Verification items for the finished model (mm, model axes). A direction names the side the tool comes from. Coordinates: 2 decimals unless noted, no trailing zeros. Write each loop counter-clockwise with the first axis right and the second up, starting at its lowest first coordinate (ties: lowest second). Pieces come first, ordered by that corner, then holes. Notation, with made-up numbers: M 74.25,40.25 L 95.25,40.25 A38 cw 95.25,78.25 Z; hole C -5,26 d1. An arc over 180 degrees is marked long. One line per item, written item: value.
```python
from build123d import *

# Parameters (mm, degrees)
SKETCH1_W           = 60
SKETCH1_H           = 20
BOSS_EXTRUDE1_DEPTH = 10
SKETCH2_R           = 1
CUT_EXTRUDE1_DEPTH  = 10
CUT_EXTRUDE4_DEPTH  = 34.166247904
SKETCH6_R           = 1.5
CUT_EXTRUDE5_DEPTH  = 46.82575695
CUT_EXTRUDE6_START  = -5
SKETCH7_R           = 3.5
CUT_EXTRUDE6_DEPTH  = 41.82575695
FILLET2_R           = 2


with BuildPart() as part:
    # Sketch1 → Boss-Extrude1 (new body)
    with BuildSketch(Plane(origin=(0, 0, 0), x_dir=(1, 0, 0), z_dir=(0, 1, 0))):
        Rectangle(SKETCH1_W, SKETCH1_H)
    extrude(amount=BOSS_EXTRUDE1_DEPTH)

    # Sketch2 → Cut-Extrude1 (cut)
    with BuildSketch(Plane(origin=(0, 10, 0), x_dir=(1, 0, 0), z_dir=(0, 1, 0))):
        with Locations(Location((-25, 4.25, 0), (0, 0, 270))):
            Circle(SKETCH2_R)
        with Locations(Location((-16.5, 4.25, 0), (0, 0, 270))):
            Circle(SKETCH2_R)
        with Locations(Location((-16.5, -4.25, 0), (0, 0, 270))):
            Circle(SKETCH2_R)
        with Locations(Location((-25, -4.25, 0), (0, 0, 270))):
            Circle(SKETCH2_R)
    extrude(amount=-CUT_EXTRUDE1_DEPTH, mode=Mode.SUBTRACT)

    # Sketch5 → Cut-Extrude4 (cut, through all)
    with BuildSketch(Plane(origin=(0, 10, 0), x_dir=(1, 0, 0), z_dir=(0, 1, 0))):
        Polygon((10, -10), (30, 10), (30, -10), align=None)
    extrude(amount=-CUT_EXTRUDE4_DEPTH, mode=Mode.SUBTRACT)

    # Sketch6 → Cut-Extrude5 (cut, through all)
    with BuildSketch(Plane(origin=(10, 0, 10), x_dir=(0.7071067811865487, 0, -0.7071067811865464), z_dir=(0.7071067811865464, 0, 0.7071067811865487))):
        with Locations((19, 5)):
            Circle(SKETCH6_R)
        with Locations((9, 5)):
            Circle(SKETCH6_R)
    extrude(amount=-CUT_EXTRUDE5_DEPTH, mode=Mode.SUBTRACT)

    # Sketch7 → Cut-Extrude6 (cut, through all)
    with BuildSketch(Plane(origin=(10, 0, 10), x_dir=(0.7071067811865487, 0, -0.7071067811865464), z_dir=(0.7071067811865464, 0, 0.7071067811865487)).offset(CUT_EXTRUDE6_START)):
        with Locations((19, 5)):
            Circle(SKETCH7_R)
        with Locations((9, 5)):
            Circle(SKETCH7_R)
    extrude(amount=-CUT_EXTRUDE6_DEPTH, mode=Mode.SUBTRACT)

    # Fillet2
    # the kernel refuses this fillet: 2 mm, written as the material it takes off along each edge
    with BuildSketch(Plane(origin=(15, 10, 10), x_dir=(0, -1, 0), z_dir=(-1, 0, 0))) as fillet2_piece_1:
        with BuildLine():
            CenterArc((FILLET2_R, -FILLET2_R), FILLET2_R, 90, 90)
            Line((0, -FILLET2_R), (0, 0))
            Line((0, 0), (FILLET2_R, 0))
        make_face()
    extrude(amount=50, mode=Mode.SUBTRACT)
    with BuildSketch(Plane(origin=(15, 0, 10), x_dir=(0, 1, 0), z_dir=(-1, 0, 0))) as fillet2_piece_2:
        with BuildLine():
            CenterArc((FILLET2_R, FILLET2_R), FILLET2_R, 180, 90)
            Line((0, FILLET2_R), (0, 0))
            Line((0, 0), (FILLET2_R, 0))
        make_face()
    extrude(amount=50, mode=Mode.SUBTRACT)
    with BuildSketch(Plane(origin=(-35, 0, -10), x_dir=(0, 0, 1), z_dir=(1, 0, 0))) as fillet2_piece_3:
        with BuildLine():
            CenterArc((FILLET2_R, -FILLET2_R), FILLET2_R, 90, 90)
            Line((0, -FILLET2_R), (0, 0))
            Line((0, 0), (FILLET2_R, 0))
        make_face()
    extrude(amount=70, mode=Mode.SUBTRACT)
    with BuildSketch(Plane(origin=(-35, 10, -10), x_dir=(0, 0, 1), z_dir=(1, 0, 0))) as fillet2_piece_4:
        with BuildLine():
            CenterArc((FILLET2_R, FILLET2_R), FILLET2_R, 180, 90)
            Line((0, FILLET2_R), (0, 0))
            Line((0, 0), (FILLET2_R, 0))
        make_face()
    extrude(amount=70, mode=Mode.SUBTRACT)


solid = part.part
```
Item 1: Access from +Z, -Z, +X, -X, +Y, -Y to the whole of each face (thin tool, end or side, straight path). Record for faces 4 (the face through (20.965, 4.271, -8.036)), 5 (the face through (-25.976, 5.07, -4.467)).
The answers:
face 4: none
face 5: +Y, -Y
Item 2: Scan lines: line 1 (X direction, y = 3, z = -7.75); line 2 (X direction, y = 4, z = 3.75); line 3 (X direction, y = 5.5, z = -5). Record each from-to range of solid material in increasing order.
The answers:
line 1: x = -30 to 0.92, 9.04 to 15.06, 20.68 to 27.75
line 2: x = -30 to -25.87, -24.13 to -17.37, -15.63 to 14.9
line 3: x = -30 to -25.66, -24.34 to -17.16, -15.84 to 2.83, 12.63 to 16.97, 17.93 to 19.87, 23.87 to 25
Item 3: Draft check along Y on faces 1 (the face through (15.63, 5.45, 0.88)), 2 (the face through (-8, 10, 0)), 3 (the face through (-25.976, 5.07, 4.033)). Enter one of: released by +Y, released by -Y, zero draft, split by the parting line, or undercut.
The answers:
face 1: undercut
face 2: released by +Y
face 3: zero draft
Item 4: Cross-section at A-A, the plane x = -16.5. Enter the section's corners in (y, z).
The answers:
outline: M 0,-8 A2 ccw 2,-10 L 8,-10 A2 ccw 10,-8 L 10,-5.25 L 0,-5.25 Z; M 0,-3.25 L 10,-3.25 L 10,3.25 L 0,3.25 Z; M 0,5.25 L 10,5.25 L 10,8 A2 ccw 8,10 L 2,10 A2 ccw 0,8 Z
Item 5: Go/stop test with flat-tipped pins: P1, Ø1.5, axis at x = -6, y = 1, coming from the +Z side; P2, Ø2, axis at x = 6, y = 6, coming from the -Z side; P3, Ø1, axis at x = 13.5, y = 2.5, coming from the +Z side; P4, Ø1.2, axis at x = -25, z = -4.25, coming from the +Y side. Record where each tip stops, or that it passes through.
The answers:
P1: stops at z = 9.98
P2: stops at z = -3.13
P3: stops at z = 7
P4: passes through
Item 6: Cross-section at B-B, the plane y = 4.25. Enter the section's corners in (x, z), and give its area (3 significant figures).
The answers:
outline: M -30,-10 L -2.11,-10 L 10.41,2.52 L 11.91,1.02 L 15.45,4.55 L 10,10 L -30,10 Z; M 7.56,-10 L 12.04,-10 L 17.48,-4.55 L 18.98,-6.05 L 22.52,-2.52 L 17.28,2.72 L 13.75,-0.82 L 15.25,-2.32 Z; M 20.82,-7.89 L 22.32,-9.39 L 21.7,-10 L 30,-10 L 24.35,-4.35 Z; hole C -25,-4.25 d2; hole C -25,4.25 d2; hole C -16.5,-4.25 d2; hole C -16.5,4.25 d2
area: 834 mm²
